from build123d import *

# Parameters (mm, degrees)
CUT_EXTRUDE_START   = 3
SKETCH_2_W          = 6
SKETCH_2_H          = 8
SKETCH_2_H_2        = 6
CUT_EXTRUDE_1_DEPTH = 1
CHAMFER_1_SIZE      = 3
SKETCH_3_R          = 1.5
CUT_EXTRUDE_4_DEPTH = 42.798624379
CHAMFER_2_SIZE      = 0.5


with BuildPart() as part:
    # 草图1 → 旋转1 (revolve)
    with BuildSketch(Plane(origin=(0, 0, 0), x_dir=(0, 0, -1), z_dir=(1, 0, 0)), mode=Mode.PRIVATE) as revolve_1_sk:
        Polygon((0, 0), (0, 3), (11.8, 3), (11.8, 13.75), (13.8, 13.75), (13.8, 3), (48.8, 3), (48.8, 0), align=None)
    revolve(revolve_1_sk.sketch.rotate(Axis((0, 0, 33.540983607), (0, 0, -1)), 90), axis=Axis((0, 0, 33.540983607), (0, 0, -1)))

    # 草图2 → 切除-拉伸1 (cut)
    with BuildSketch(Plane(origin=(0, 0, 0), x_dir=(1, 0, 0), z_dir=(0, 1, 0)).offset(CUT_EXTRUDE_START)):
        with Locations((0, 33.6)):
            Rectangle(SKETCH_2_W, SKETCH_2_H)
        with Locations((0, 3)):
            Rectangle(SKETCH_2_W, SKETCH_2_H_2)
    extrude(amount=-CUT_EXTRUDE_1_DEPTH, mode=Mode.SUBTRACT)

    # 倒角1
    chamfer_1_edges = [part.edges().sort_by_distance(p)[0] for p in [
        (-3, 0, -11.8),
    ]]
    chamfer(chamfer_1_edges, length=CHAMFER_1_SIZE)

    # 草图3 → 切除-拉伸4 (cut, through all)
    with BuildSketch(Plane.XY.offset(-11.8)):
        with Locations((5.75, -9.959292144)):
            Circle(SKETCH_3_R)
        with Locations((-11.5, 0)):
            Circle(SKETCH_3_R)
        with Locations((5.75, 9.959292144)):
            Circle(SKETCH_3_R)
    extrude(amount=-CUT_EXTRUDE_4_DEPTH, mode=Mode.SUBTRACT)

    # 倒角2
    chamfer_2_edges = [part.edges().sort_by_distance(p)[0] for p in [
        (-1.070466269, -2.802517077, 0),
        (-3, 0, -48.8),
    ]]
    chamfer(chamfer_2_edges, length=CHAMFER_2_SIZE)


solid = part.part
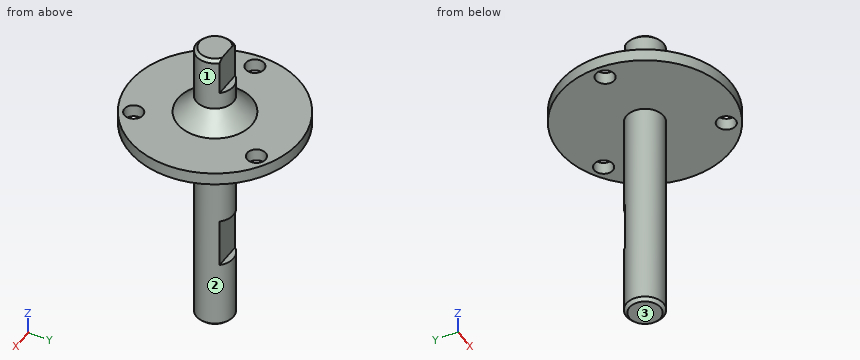
Work out the finished part from the listing and answer in its coordinate system (mm). Face numbers are marked on the shaded views. A direction names the side the tool comes from. Give positions to 0.01 mm unless a question says otherwise; leave off trailing zeros. Loops run counter-clockwise (first coordinate to the right, second up) from the corner with the lowest first, then second, coordinate; pieces in that order, holes last. Notation, with made-up numbers: M 80.5,-33.75 L 103.5,-33.75 A11 cw 103.5,-21.75 Z; hole C 29.25,-15.75 d4. An arc over 180 degrees is marked long. Use CSV: the item, a comma, the result in double quotes.
1) Find section D-D on z = -24. Write down the section's boundary in (x, y).
Answer:
outline,"C 0,0 d6"
2) Consider L1, parallel to Y at x = 5.75, z = -12.25; L2, parallel to Z at x = 4, y = -6; L3, parallel to X at y = -1.75, z = -41.5. Determine where each line is inside the solid, lowest interval first.
Answer:
L1,"-12.49 to -11.46, -8.46 to 8.46, 11.46 to 12.49"
L2,"-13.8 to -11.8"
L3,"-2.44 to 2.44"
3) Which of the six approach directions +Z, -Z, +X, -X, +Y, -Y give full straight-line access (tool end or side, diameter ignored) to the marked faces 1, 2 and 3?
Answer:
face 1,"+Z"
face 2,"-Z"
face 3,"-Z, +X, -X, +Y, -Y"
4) Find section B-B on x = -11.5. Write down the section's boundary in (y, z).
Answer:
outline,"M -7.54,-13.8 L -1.5,-13.8 L -1.5,-11.8 L -7.54,-11.8 Z; M 1.5,-13.8 L 7.54,-13.8 L 7.54,-11.8 L 1.5,-11.8 Z"
5) Find section C-C on x = 0. Write down the section's boundary in (y, z).
Answer:
outline,"M -13.75,-13.8 L -3,-13.8 L -3,-48.3 L -2.5,-48.8 L 2.5,-48.8 L 3,-48.3 L 3,-37.6 L 2,-37.6 L 2,-29.6 L 3,-29.6 L 3,-13.8 L 13.75,-13.8 L 13.75,-11.8 L 6,-11.8 L 3,-8.8 L 3,-6 L 2,-6 L 2,0 L -2.5,0 L -3,-0.5 L -3,-8.8 L -6,-11.8 L -13.75,-11.8 Z"
6) Given P1, Ø5, axis at x = -0.5, z = -2, coming from the +Y side; P2, Ø5, axis at x = -11.5, y = 0, coming from the +Z side; P3, Ø1.8, axis at x = 5.75, y = 9.96, coming from the -Z side; P4, Ø0.8, axis at x = 0.5, y = 2.5, coming from the +Z side, each flat-ended and moving along its own axis, determine where each tip first touches the part or whether it passes through.
Answer:
P1,"y = 2"
P2,"z = -11.8"
P3,"through"
P4,"z = -6"
7) Find section A-A on y = 0. Write down the section's boundary in (x, z), plus the area to 3 significant figures.
Answer:
outline,"M -13.75,-13.8 L -13,-13.8 L -13,-11.8 L -13.75,-11.8 Z; M -10,-13.8 L -3,-13.8 L -3,-48.3 L -2.5,-48.8 L 2.5,-48.8 L 3,-48.3 L 3,-13.8 L 13.75,-13.8 L 13.75,-11.8 L 6,-11.8 L 3,-8.8 L 3,-0.5 L 2.5,0 L -2.5,0 L -3,-0.5 L -3,-8.8 L -6,-11.8 L -10,-11.8 Z"
area,"338 mm^2"
